Verification items for the finished model (mm, model axes). Face numbers are marked on the shaded views. A direction names the side the tool comes from. Give positions to 0.01 mm unless a question says otherwise; leave off trailing zeros. Write each loop counter-clockwise with the first axis right and the second up, starting at its lowest first coordinate (ties: lowest second). Pieces come first, ordered by that corner, then holes. Notation, with made-up numbers: (80.5, 65.25) - (105.5, 65.25) arc R20 ccw to (105.5, 79.25) - close; hole circle Ø8 at (69, 86.5). An arc over 180 degrees is marked (long way). Answer as a JSON object with one key per item and string values. Group by question number.
Item 1: Sectioned sample at A-A, the plane y = 0. Record the boundary of the cut face in (x, z), and give its area (3 significant figures).
Item 2: Sectioned sample at D-D, the plane x = 0. Count the separate pieces of the cut face and the enclosed holes in it, and give its area (3 significant figures).
Item 3: Go/stop test with flat-tipped pins: pin 1 (1 mm diameter, centred on y = 21.5, z = 7, fed in from -X); pin 2 (5 mm diameter, centred on x = -18.94, z = 14.29, fed in from +Y); pin 3 (3 mm diameter, centred on y = 3.5, z = 13, fed in from -X). Record where each tip stops, or that it passes through.
Item 4: Tool access check on the marked faces 4, 5 and 6. Record the directions out of +Z, -Z, +X, -X, +Y, -Y that give a thin tool (end or side, any length) a straight path to the whole face; none if there is none.
Item 5: Draft check along X on the marked faces 1, 2 and 3. Enter one of: +X half, -X half, draft (parallel to the pull), parting line (faces both ways), or undercut.
Item 6: Scan lines: line 1 along Y through (x, z) = (-14.75, 14) (3 decimals); line 2 along X through (y, z) = (1.5, 17.5); line 3 along X through (y, z) = (16.5, 3). Record each from-to range of solid material in increasing order. Write a range as [from, to].
Item 7: Sectioned sample at C-C, the plane x = -18. Record the boundary of the cut face in (y, z) (3 decimals), and give its area (3 significant figures).
```python
from build123d import *

# Parameters (mm, degrees)
BOSS_EXTRUDE1_DEPTH     = 19.05
F_6_CLEARANCE_HOLE1_D   = 3.7973
FILLET1_R               = 3.175
E_0_25_DIAMETER_HOLE1_D = 3.2639
E_0_25_DIAMETER_HOLE2_D = 3.2639


with BuildPart() as part:
    # Sketch1 → Boss-Extrude1 (new body)
    with BuildSketch(Plane.XY):
        with BuildLine():
            Line((-7.332348419, 12.7), (0.605151581, 26.448153285))
            Line((0.605151581, 26.448153285), (3.354782238, 24.860653285))
            Line((3.354782238, 24.860653285), (-1.833087105, 15.875))
            Line((-1.833087105, 15.875), (5.499261314, 3.175))
            ThreePointArc((5.499261314, 3.175), (3.175, -5.499261314), (-5.499261314, -3.175))
            Line((-5.499261314, -3.175), (-12.831609733, 9.525))
            Line((-12.831609733, 9.525), (-23.207348419, 9.525))
            Line((-23.207348419, 9.525), (-23.207348419, 12.7))
            Line((-23.207348419, 12.7), (-7.332348419, 12.7))
        make_face()
    extrude(amount=BOSS_EXTRUDE1_DEPTH)

    # #6 Clearance Hole1 (through all)
    with Locations(Plane(origin=(0, 0, 0), x_dir=(-1, 0, 0), z_dir=(0, 0, -1))):
        with Locations((0, 0)):
            Hole(F_6_CLEARANCE_HOLE1_D / 2)

    # Fillet1
    fillet1_edges = [part.edges().sort_by_distance(p)[0] for p in [
        (-1.833087105, 15.875, 9.525),
        (-12.831609733, 9.525, 9.525),
    ]]
    fillet(fillet1_edges, radius=FILLET1_R)

    # E (0.25) Diameter Hole1 (through all)
    with Locations(Plane(origin=(-8.248891971, 4.7625, 0), x_dir=(0, 0, -1), z_dir=(0.86602540378444, -0.49999999999999784, 0))):
        with Locations((-4.7625, 18.936022628), (-14.2875, 18.936022628)):
            Hole(E_0_25_DIAMETER_HOLE1_D / 2)

    # E (0.25) Diameter Hole2 (through all)
    with Locations(Plane(origin=(-18.936022628, 9.525, 14.2875), x_dir=(-1, 0, 0), z_dir=(0, -1, 0))):
        with Locations((0, 0), (0, 9.525)):
            Hole(E_0_25_DIAMETER_HOLE2_D / 2)


solid = part.part
```
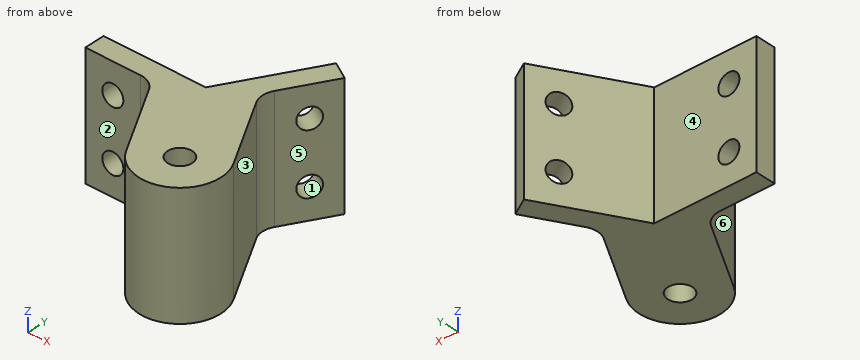
Geometry check:
{
 "1": {"outline": "(-7.33, 0) - (-1.9, 0) - (-1.9, 19.05) - (-7.33, 19.05) - close; (1.9, 0) - (6.35, 0) - (6.35, 19.05) - (1.9, 19.05) - close", "area": "188 mm^2"},
 "2": {"separate pieces": "3", "enclosed holes": "2", "area": "392 mm^2"},
 "3": {"pin 1": "x = -2.54", "pin 2": "y = 12.7", "pin 3": "x = -10.22"},
 "4": {"face 4": "+Z, -Z, -X, +Y", "face 5": "+Z, -Z, +X", "face 6": "+Z, -Z, -X, -Y"},
 "5": {"face 1": "undercut", "face 2": "draft", "face 3": "+X half"},
 "6": {"line 1": "[9.525, 12.7]", "line 2": "[-8.2, -1.16], [1.16, 6.17]", "line 3": "[-5.14, -1.28]"},
 "7": {"outline": "(9.525, 0) - (12.7, 0) - (12.7, 3.426) - (9.525, 3.426) - close; (9.525, 6.099) - (12.7, 6.099) - (12.7, 12.951) - (9.525, 12.951) - close; (9.525, 15.624) - (12.7, 15.624) - (12.7, 19.05) - (9.525, 19.05) - close", "area": "43.5 mm^2"}
}
